from build123d import *

# Parameters (mm, degrees)
SKETCH1_W           = 50.8
SKETCH1_H           = 49.022
BOSS_EXTRUDE2_DEPTH = 16.51
FILLET1_R           = 2.032
SHELL2_T            = -1.27
SKETCH4_W           = 3.556
SKETCH4_H           = 10.16
CUT_EXTRUDE2_DEPTH  = 1.27
SKETCH7_W           = 3.2520636
SKETCH7_H           = 1.903459875
BOSS_EXTRUDE5_DEPTH = 2.286
FILLET6_R           = 1.016
SKETCH8_W           = 1.778
SKETCH8_H           = 3.302
BOSS_EXTRUDE6_DEPTH = 2.286
FILLET7_R           = 1.016
SKETCH9_W           = 3.302
SKETCH9_H           = 1.778
BOSS_EXTRUDE7_DEPTH = 2.286
FILLET8_R           = 1.016


with BuildPart() as part:
    # Sketch1 → Boss-Extrude2 (new body)
    with BuildSketch(Plane.XY):
        with Locations((25.4, 24.511)):
            Rectangle(SKETCH1_W, SKETCH1_H)
    extrude(amount=BOSS_EXTRUDE2_DEPTH)

    # Fillet1
    fillet1_edges = [part.edges().sort_by_distance(p)[0] for p in [
        (0, 0, 8.255),
        (50.8, 0, 8.255),
        (50.8, 49.022, 8.255),
        (0, 49.022, 8.255),
    ]]
    fillet(fillet1_edges, radius=FILLET1_R)

    # Shell2
    shell2_openings = [part.faces().sort_by_distance(p)[0] for p in [
        (25.4, 24.511, 16.51),
    ]]
    offset(amount=SHELL2_T, openings=shell2_openings, kind=Kind.INTERSECTION)

    # Sketch4 → Cut-Extrude2 (cut)
    with BuildSketch(Plane.ZY):
        with Locations((6.35, 38.862)):
            Rectangle(SKETCH4_W, SKETCH4_H)
    extrude(amount=-CUT_EXTRUDE2_DEPTH, mode=Mode.SUBTRACT)

    # Sketch7 → Boss-Extrude5 (add)
    with BuildSketch(Plane(origin=(0, 49.022, 0), x_dir=(1, 0, 0), z_dir=(0, 1, 0))):
        with Locations((23.095521807, -6.285729938)):
            Rectangle(SKETCH7_W, SKETCH7_H)
    extrude(amount=-BOSS_EXTRUDE5_DEPTH)

    # Fillet6
    fillet6_edges = [part.edges().sort_by_distance(p)[0] for p in [
        (23.095521807, 46.736, 7.237459875),
    ]]
    fillet(fillet6_edges, radius=FILLET6_R - 0.0001)  # a hair under: the kernel refuses the full size

    # Sketch8 → Boss-Extrude6 (add)
    with BuildSketch(Plane(origin=(50.8, 0, 0), x_dir=(0, 0, -1), z_dir=(1, 0, 0))):
        with Locations((-6.223, 26.013260114)):
            Rectangle(SKETCH8_W, SKETCH8_H)
    extrude(amount=-BOSS_EXTRUDE6_DEPTH)

    # Fillet7
    fillet7_edges = [part.edges().sort_by_distance(p)[0] for p in [
        (48.514, 26.013260114, 7.112),
    ]]
    fillet(fillet7_edges, radius=FILLET7_R - 0.0001)  # a hair under: the kernel refuses the full size

    # Sketch9 → Boss-Extrude7 (add)
    with BuildSketch(Plane.XZ):
        with Locations((26.526394694, 6.223)):
            Rectangle(SKETCH9_W, SKETCH9_H)
    extrude(amount=-BOSS_EXTRUDE7_DEPTH)

    # Fillet8
    fillet8_edges = [part.edges().sort_by_distance(p)[0] for p in [
        (26.526394694, 2.286, 7.112),
    ]]
    fillet(fillet8_edges, radius=FILLET8_R - 0.0001)  # a hair under: the kernel refuses the full size


solid = part.part
Geometry: final body of the model. Coordinates: model frame, mm. A direction names the side the tool comes from. Coordinates: 2 decimals unless noted, no trailing zeros. Loops run counter-clockwise (first coordinate to the right, second up) from the corner with the lowest first, then second, coordinate; pieces in that order, holes last. Notation, with made-up numbers: (2.5, 48) - (16.5, 48) arc R19 cw to (16.5, 80) - close; hole circle Ø5 at (10, 72). An arc over 180 degrees is marked (long way). Put each result on its own line as item: value. Start each with the question number.
Q1. Cut plane A-A, the plane z = 12.75. Return loops of the section in (x, y), and give its area (3 significant figures).
Q2. Cut plane D-D, the plane y = 12. Return loops of the section in (x, z), and give its area (3 significant figures).
Q3. Cut plane B-B, the plane y = 34.5. Return loops of the section in (x, z).
Q4. Pin query (flat end, axial travel): pin 1 Ø0.5 at (y, z) = (47.5, 6) entering from -X; pin 2 Ø1.4 at (x, z) = (1, 6.5) entering from +Y; pin 3 Ø10 at (x, y) = (34, 31) entering from +Z. Return the tip coordinate at first contact, or that it passes through.
Q5. Pull-direction query (Z, two-part tool) for faces 1 (the flat face through (25, 49.022, 8)), 2 (the flat face through (23, 1, 16.51)), 3 (the flat face through (1, 39, 8.128)); classes: released by +Z, released by -Z, zero draft, split by the parting line, or undercut.
Q6. Set-up query: faces 4 (the flat face through (0, 24, 8)), 5 (the flat face through (1.27, 24, 9)), 6 (the flat face through (1, 33.782, 6)). Return all of +Z, -Z, +X, -X, +Y, -Y with unobstructed straight access to the full face (end or side cutting, diameter ignored); none if empty.
Q7. Line query: line 1 (Y direction, x = 23, z = 4); line 2 (X direction, y = 13.5, z = 9.75); line 3 (Z direction, x = 5, y = 22). Output: solid intervals per line, ascending.
Filled sheet:
1. outline: (0, 2.03) arc R2.03 ccw to (2.03, 0) - (48.77, 0) arc R2.03 ccw to (50.8, 2.03) - (50.8, 46.99) arc R2.03 ccw to (48.77, 49.02) - (2.03, 49.02) arc R2.03 ccw to (0, 46.99) - close; hole (1.27, 2.03) arc R0.76 ccw to (2.03, 1.27) - (48.77, 1.27) arc R0.76 ccw to (49.53, 2.03) - (49.53, 46.99) arc R0.76 ccw to (48.77, 47.75) - (2.03, 47.75) arc R0.76 ccw to (1.27, 46.99) - close
1. area: 244 mm²
2. outline: (0, 0) - (50.8, 0) - (50.8, 16.51) - (49.53, 16.51) - (49.53, 1.27) - (1.27, 1.27) - (1.27, 16.51) - (0, 16.51) - close
2. area: 103 mm²
3. outline: (0, 0) - (50.8, 0) - (50.8, 16.51) - (49.53, 16.51) - (49.53, 1.27) - (1.27, 1.27) - (1.27, 4.57) - (0, 4.57) - close; (0, 8.13) - (1.27, 8.13) - (1.27, 16.51) - (0, 16.51) - close
4. pin 1: x = 0.02
4. pin 2: y = 48.99
4. pin 3: z = 1.27
5. face 1: zero draft
5. face 2: released by +Z
5. face 3: undercut
6. face 4: +Z, -Z, -X, +Y, -Y
6. face 5: +Z
6. face 6: -X
7. line 1: 0 to 1.27, 47.75 to 49.02
7. line 2: 0 to 1.27, 49.53 to 50.8
7. line 3: 0 to 1.27
